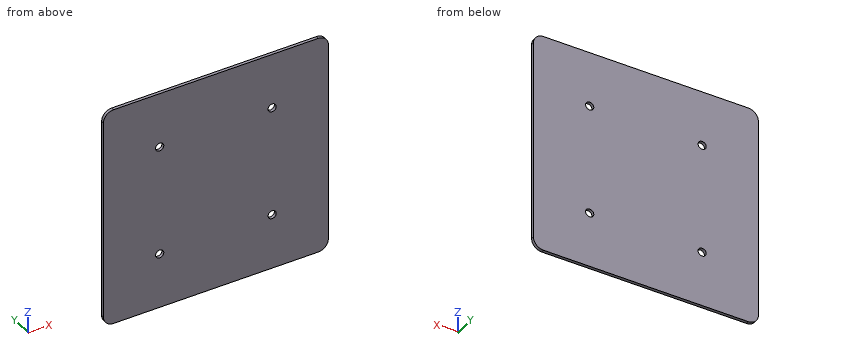
from build123d import *

# Parameters (mm, degrees)
SKETCH_1_W               = 88
SKETCH_1_H               = 88
EXTRUDE_1_DEPTH          = 1.2
FILLET_1_R               = 4
SKETCH_2_R               = 1.6
CUT_EXTRUDE_1_DEPTH      = 10
CUT_EXTRUDE_1_DEPTH_BACK = 2.2


with BuildPart() as part:
    # 草图1 → 凸台-拉伸1 (new body)
    with BuildSketch(Plane(origin=(0, 0, 0), x_dir=(1, 0, 0), z_dir=(0, 1, 0))):
        with Locations((44, -44)):
            Rectangle(SKETCH_1_W, SKETCH_1_H)
    extrude(amount=EXTRUDE_1_DEPTH)

    # 圆角1
    fillet_1_edges = [part.edges().sort_by_distance(p)[0] for p in [
        (0, 0.6, 0),
        (88, 0.6, 0),
        (88, 0.6, 88),
        (0, 0.6, 88),
    ]]
    fillet(fillet_1_edges, radius=FILLET_1_R)

    # 草图2 → 切除-拉伸1 (cut, two sides)
    with BuildSketch(Plane(origin=(0, 1.2, 0), x_dir=(1, 0, 0), z_dir=(0, 1, 0))) as cut_extrude_1_sk:
        with Locations((22, -22)):
            Circle(SKETCH_2_R)
        with Locations((66, -22)):
            Circle(SKETCH_2_R)
        with Locations((66, -66)):
            Circle(SKETCH_2_R)
        with Locations((22, -66)):
            Circle(SKETCH_2_R)
    extrude(amount=CUT_EXTRUDE_1_DEPTH, mode=Mode.SUBTRACT)
    extrude(cut_extrude_1_sk.sketch, amount=-CUT_EXTRUDE_1_DEPTH_BACK, mode=Mode.SUBTRACT)


solid = part.part
Geometry check sheet. Reference: the model listing, model coordinates, mm. Give positions to 0.01 mm unless a question says otherwise; leave off trailing zeros. Loops run counter-clockwise (first coordinate to the right, second up) from the corner with the lowest first, then second, coordinate; pieces in that order, holes last.
(1) Depth check by flat-ended pin: pin 1 Ø3 at (x, z) = (22, 66) entering from -Y. Enter the tip coordinate at first touch or a pass-through.
From the geometry:
pin 1: passes through
(2) Section check B-B on x = 66. Record the cut outline in (y, z), then the cut area to 3 significant figures.
From the geometry:
outline: (0, 0) - (1.2, 0) - (1.2, 20.4) - (0, 20.4) - close; (0, 23.6) - (1.2, 23.6) - (1.2, 64.4) - (0, 64.4) - close; (0, 67.6) - (1.2, 67.6) - (1.2, 88) - (0, 88) - close
area: 97.9 mm2
(3) Thickness scan on L1, parallel to Z at x = 22, y = 0.6; L2, parallel to Z at x = 23, y = 1.05. Record the ranges inside material, lowest first.
From the geometry:
L1: z = 0 to 20.4, 23.6 to 64.4, 67.6 to 88
L2: z = 0 to 20.75, 23.25 to 64.75, 67.25 to 88
(4) Section check A-A on z = 66. Record the cut outline in (x, y), then the cut area to 3 significant figures.
From the geometry:
outline: (0, 0) - (20.4, 0) - (20.4, 1.2) - (0, 1.2) - close; (23.6, 0) - (64.4, 0) - (64.4, 1.2) - (23.6, 1.2) - close; (67.6, 0) - (88, 0) - (88, 1.2) - (67.6, 1.2) - close
area: 97.9 mm2
